Read the model definition and answer for the solid it produces. Units are mm, in the model's axes. Face numbers are marked on the shaded views. A direction names the side the tool comes from. Give positions to 0.01 mm unless a question says otherwise; leave off trailing zeros. Write each loop counter-clockwise with the first axis right and the second up, starting at its lowest first coordinate (ties: lowest second). Pieces come first, ordered by that corner, then holes. Notation, with made-up numbers: (83, 1) -> (130, 1) arc R6 cw to (130, 6) -> close; hole circle Ø1 at (49, 60.25). An arc over 180 degrees is marked (long way). Answer as CSV lines item,"result". Start each with the question number.
1. The part is cut by section D-D, the plane z = -7.5. Give the number of separate pieces and of enclosed holes in the cut face, and give its area (3 significant figures).
2. For a pull along Y with two mould halves and no side action, classify the marked faces 6, 7 and 8 as pulls with the +Y half, pulls with the -Y half, needs draft (parallel to the pull), parting line crosses it, or undercut.
3. Find the intervals of material crossed by line 1 (Y direction, x = 5, z = 4.75); line 2 (Z direction, x = 13.5, y = 3.75); line 3 (Z direction, x = 6, y = -5), in increasing order.
4. The part is cut by section A-A, the plane x = -11.5. Determine the outline of the cut face in (y, z), and give its area (3 significant figures).
5. The part is cut by section C-C, the plane y = 0. Determine the outline of the cut face in (x, z), and give its area (3 significant figures).
6. A tool of negligible diameter and unlimited length cuts with its end or side. For the marked faces 1, 2, 3, 4 and 5, from which of +Z, -Z, +X, -X, +Y, -Y can it reach the whole face along a straight path? Write none if from no direction.
7. The part is cut by section B-B, the plane z = 3. Determine the outline of the cut face in (x, y), and give its area (3 significant figures).
8. Given pin 1 (5 mm diameter, centred on x = -1, z = 5.5, fed in from +Y); pin 2 (6 mm diameter, centred on y = 1, z = -7, fed in from -X); pin 3 (6.5 mm diameter, centred on x = 0.5, z = 5.5, fed in from -Y); pin 4 (2.5 mm diameter, centred on x = 12.495, y = 0, fed in from +Z), each flat-ended and moving along its own axis, determine where each tip first touches the part or whether it passes through.
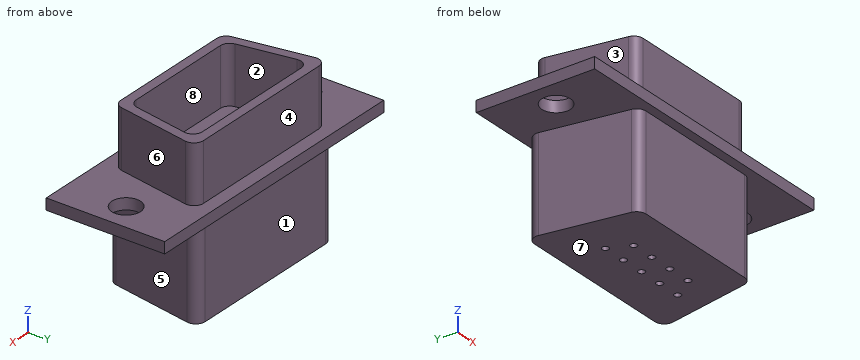
from build123d import *

# Parameters (mm, degrees)
SKETCH_1_W             = 30.8
SKETCH_1_H             = 12.6
EXTRUDE_1_DEPTH        = 1.2
EXTRUDE_2_DEPTH        = 6.1
EXTRUDE_3_DEPTH        = 10
HOLE_WIZARD_0000_1_D   = 0.7112
HOLE_WIZARD_0000_2_D   = 0.7112
PATTERN_LINEAR_1_COUNT = 5
PATTERN_LINEAR_1_PITCH = 2.54
PATTERN_LINEAR_2_COUNT = 4
PATTERN_LINEAR_2_PITCH = 2.54
HOLE_WIZARD_3_2_D      = 3.048
FILLET_1_R             = 1


with BuildPart() as part:
    # ｽｹｯﾁ1 → ﾎﾞｽ - 押し出し1 (new body)
    with BuildSketch(Plane.XY):
        Rectangle(SKETCH_1_W, SKETCH_1_H)
    extrude(amount=EXTRUDE_1_DEPTH)

    # ｽｹｯﾁ2 → ﾎﾞｽ - 押し出し2 (add)
    with BuildSketch(Plane.XY.offset(1.2)):
        Polygon((-9.321753593, 4.91), (9.321753593, 4.91), (7.590222642, -4.91), (-7.590222642, -4.91), align=None)
        Polygon((-6.751123011, -3.91), (6.751123011, -3.91), (8.13, 3.91), (-8.13, 3.91), align=None, mode=Mode.SUBTRACT)
    extrude(amount=EXTRUDE_2_DEPTH)

    # ｽｹｯﾁ3 → ﾎﾞｽ - 押し出し3 (add)
    with BuildSketch(Plane(origin=(0, 0, 0), x_dir=(-1, 0, 0), z_dir=(0, 0, -1))):
        Polygon((-7.763301306, -5.35), (7.763301306, -5.35), (9.65, 5.35), (-9.65, 5.35), align=None)
    extrude(amount=EXTRUDE_3_DEPTH)

    # #0000 すきま穴1 (through all)
    with Locations(Plane(origin=(-4.225439316, 1.008007938, 1.2), x_dir=(1, 0, 0), z_dir=(0, 0, 1))):
        with Locations((0, 0)):
            hole_wizard_0000_1 = Hole(HOLE_WIZARD_0000_1_D / 2)

    # #0000 すきま穴2 (through all)
    with Locations(Plane(origin=(-3.168321124, -1.202810505, 1.2), x_dir=(1, 0, 0), z_dir=(0, 0, 1))):
        with Locations((0, 0)):
            hole_wizard_0000_2 = Hole(HOLE_WIZARD_0000_2_D / 2)

    # 直線ﾊﾟﾀｰﾝ1: #0000 すきま穴1 ×5
    with Locations(*[(i * PATTERN_LINEAR_1_PITCH, 0, 0) for i in range(1, PATTERN_LINEAR_1_COUNT)]):
        add(hole_wizard_0000_1, mode=Mode.SUBTRACT)

    # 直線ﾊﾟﾀｰﾝ2: #0000 すきま穴2 ×4
    with Locations(*[(i * PATTERN_LINEAR_2_PITCH, 0, 0) for i in range(1, PATTERN_LINEAR_2_COUNT)]):
        add(hole_wizard_0000_2, mode=Mode.SUBTRACT)

    # #3 すきま穴2 (through all)
    with Locations(Plane(origin=(-12.495, 0, 1.2), x_dir=(1, 0, 0), z_dir=(0, 0, 1))):
        with Locations((0, 0), (24.99, 0)):
            Hole(HOLE_WIZARD_3_2_D / 2)

    # ﾌｨﾚｯﾄ1
    fillet_1_edges = [part.edges().sort_by_distance(p)[0] for p in [
        (-9.321753593, 4.91, 4.25),
        (-7.590222642, -4.91, 4.25),
        (7.590222642, -4.91, 4.25),
        (9.321753593, 4.91, 4.25),
        (8.13, 3.91, 4.25),
        (-8.13, 3.91, 4.25),
        (-6.751123011, -3.91, 4.25),
        (6.751123011, -3.91, 4.25),
        (-7.763301306, -5.35, -5),
        (-9.65, 5.35, -5),
        (9.65, 5.35, -5),
        (7.763301306, -5.35, -5),
    ]]
    fillet(fillet_1_edges, radius=FILLET_1_R)


solid = part.part
Results found:
1,separate pieces,"1"
1,enclosed holes,"9"
1,area,"182 mm²"
2,face 6,"pulls with the -Y half"
2,face 7,"needs draft"
2,face 8,"undercut"
3,line 1,"y = -4.91 to -3.91, 3.91 to 4.91"
3,line 2,"z = 0 to 1.2"
3,line 3,"z = -10 to 1.2"
4,outline,"(-6.3, 0) -> (-1.15, 0) -> (-1.15, 1.2) -> (-6.3, 1.2) -> close; (1.15, 0) -> (6.3, 0) -> (6.3, 1.2) -> (1.15, 1.2) -> close"
4,area,"12.3 mm²"
5,outline,"(-15.4, 0) -> (-14.02, 0) -> (-14.02, 1.2) -> (-15.4, 1.2) -> close; (-10.97, 0) -> (-8.71, 0) -> (-8.71, -10) -> (8.71, -10) -> (8.71, 0) -> (10.97, 0) -> (10.97, 1.2) -> (8.46, 1.2) -> (8.46, 7.3) -> (7.44, 7.3) -> (7.44, 1.2) -> (-7.44, 1.2) -> (-7.44, 7.3) -> (-8.46, 7.3) -> (-8.46, 1.2) -> (-10.97, 1.2) -> close; (14.02, 0) -> (15.4, 0) -> (15.4, 1.2) -> (14.02, 1.2) -> close"
5,area,"216 mm²"
6,face 1,"-Z, +X, -X, +Y"
6,face 2,"+Z"
6,face 3,"+Z, -X, -Y"
6,face 4,"+Z, +X, -X, +Y"
6,face 5,"-Z, +X, -Y"
7,outline,"(-9.11, 3.74) -> (-7.74, -4.08) arc R1 ccw to (-6.75, -4.91) -> (6.75, -4.91) arc R1 ccw to (7.74, -4.08) -> (9.11, 3.74) arc R1 ccw to (8.13, 4.91) -> (-8.13, 4.91) arc R1 ccw to start; hole (-7.92, 2.74) -> (-6.9, -3.08) arc R1 ccw to (-5.91, -3.91) -> (5.91, -3.91) arc R1 ccw to (6.9, -3.08) -> (7.92, 2.74) arc R1 ccw to (6.94, 3.91) -> (-6.94, 3.91) arc R1 ccw to start"
7,area,"49.7 mm²"
8,pin 1,"stops at y = 4.91"
8,pin 2,"stops at x = -9.41"
8,pin 3,"stops at y = -4.91"
8,pin 4,"passes through"
